Verification items for this drawing (mm, ordinates from the low corner). A direction names the side the tool comes from. Give positions to 0.01 mm unless a question says otherwise; leave off trailing zeros. Order: outer loops, then holes, each group sorted by start corner. A loop starts at its lowest first (then second) coordinate and runs counter-clockwise, first axis right, second up.
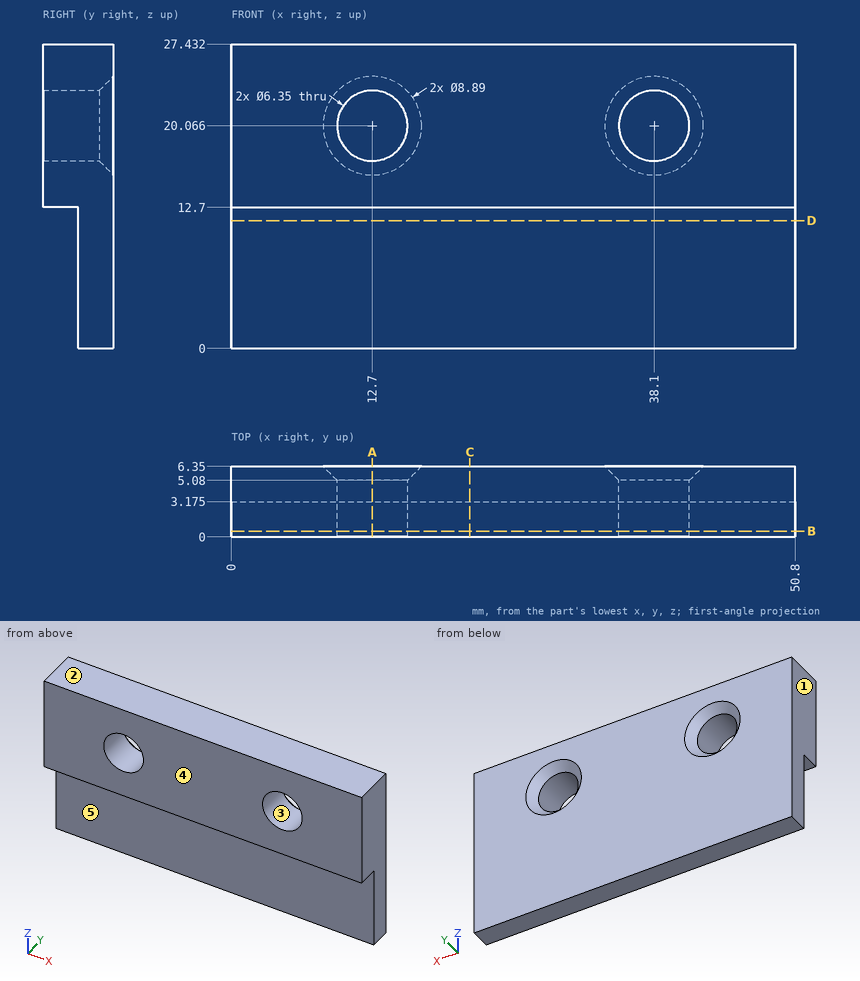
Q1. Release check for a two-part mould opening along Z. For the marked faces 1, 2 and 3 record: pulls with the +Z half, pulls with the -Z half, needs draft (parallel to the pull), parting line crosses it, or undercut.
Q2. Gauge pin test, flat ends, axial feed: P1, Ø8.5, axis at x = 12.7, z = 20.066, coming from the +Y side (3 decimals); P2, Ø10, axis at x = 37.5, z = 7.5, coming from the -Y side (3 decimals); P3, Ø1, axis at x = 37.5, y = 2, coming from the -Z side. Record the tip position at first contact, or that the pin passes through.
Q3. Cross-section at B-B, the plane y = 0.5. Record the boundary of the cut face in (x, z) (3 decimals), and give its area (3 significant figures).
Q4. Access from +Z, -Z, +X, -X, +Y, -Y to the whole of each face (thin tool, end or side, straight path). Record for the marked faces 4 and 5.
Q5. Cross-section at C-C, the plane x = 21.5. Record the boundary of the cut face in (y, z) (3 decimals).
Q6. Thickness scan on L1, parallel to Z at x = 38.1, y = 1.4; L2, parallel to X at y = 1.25, z = 19.25; L3, parallel to X at y = 4.5, z = 22.75. Record the ranges inside material, lowest first.
Q7. Cross-section at D-D, the plane z = 11.5. Record the boundary of the cut face in (x, y) (3 decimals), and give its area (3 significant figures).
Q8. Cross-section at A-A, the plane x = 12.7. Record the boundary of the cut face in (y, z) (3 decimals).
Answers follow:
1. face 1: needs draft
1. face 2: pulls with the +Z half
1. face 3: undercut
2. P1: stops at y = 6.155
2. P2: stops at y = 3.175
2. P3: stops at z = 12.7
3. outline: (0, 12.7) - (50.8, 12.7) - (50.8, 27.432) - (0, 27.432) - close; hole circle Ø6.35 at (12.7, 20.066); hole circle Ø6.35 at (38.1, 20.066)
3. area: 685 mm2
4. face 4: +Z, -Z, +X, -X, -Y
4. face 5: -Z, +X, -X, -Y
5. outline: (0, 12.7) - (3.175, 12.7) - (3.175, 0) - (6.35, 0) - (6.35, 27.432) - (0, 27.432) - close
6. L1: z = 12.7 to 16.89, 23.24 to 27.43
6. L2: x = 0 to 9.63, 15.77 to 35.03, 41.17 to 50.8
6. L3: x = 0 to 11, 14.4 to 36.4, 39.8 to 50.8
7. outline: (0, 3.175) - (50.8, 3.175) - (50.8, 6.35) - (0, 6.35) - close
7. area: 161 mm2
8. outline: (0, 12.7) - (3.175, 12.7) - (3.175, 0) - (6.35, 0) - (6.35, 15.621) - (5.08, 16.891) - (0, 16.891) - close; (0, 23.241) - (5.08, 23.241) - (6.35, 24.511) - (6.35, 27.432) - (0, 27.432) - close
